Input: part model. Units: mm. Frame: model coordinates. Give positions to 0.01 mm unless a question says otherwise; leave off trailing zeros. Write each loop counter-clockwise with the first axis right and the second up, starting at its lowest first coordinate (ties: lowest second). Pieces come first, ordered by that corner, then holes.
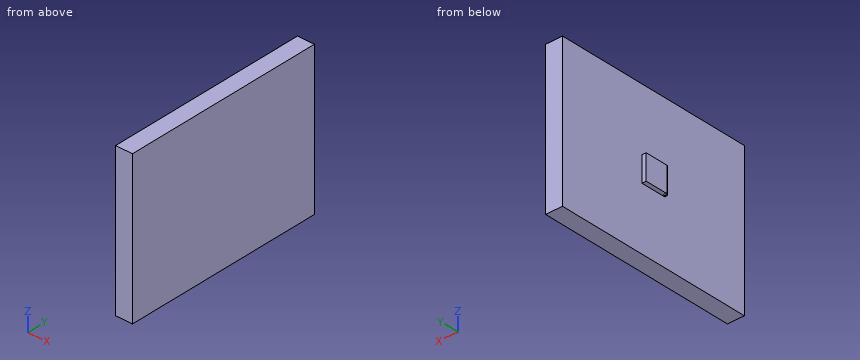
```python
from build123d import *

# Parameters (mm, degrees)
F0_W     = 304.8
F0_H     = 228.6
F1_DEPTH = 25.4
F3_DEPTH = 19.05
F5_D     = 3.175
F6_R     = 3.175


with BuildPart() as f1:
    # F0 (on Right) → F1 (new body)
    with BuildSketch(Plane.YZ):
        Rectangle(F0_W, F0_H)
    extrude(amount=F1_DEPTH)

    # F2 (on Front) → F3 (join, symmetric)
    with BuildSketch(Plane.XZ):
        Polygon((0, -19.05), (0, 19.05), (-3.175, 19.05), (-6.35, 19.05), (-6.35, -19.05), (-3.175, -19.05), align=None)
    extrude(amount=F3_DEPTH, both=True)

    # F5 (through all)
    with Locations(Plane.XY.offset(19.05)):
        with Locations((-3.175, -15.875)):
            Hole(F5_D / 2)

    # F6
    f6_edges = [f1.edges().sort_by_distance(p)[0] for p in [
        (-6.35, -19.05, 0),
    ]]
    fillet(f6_edges, radius=F6_R)


solid = f1.part
```
Q1. Pin query (flat end, axial travel): pin 1 (7 mm diameter, centred on x = -4.5, y = -9.5, fed in from +Z); pin 2 (3 mm diameter, centred on x = -4, z = 0.5, fed in from +Y); pin 3 (4 mm diameter, centred on y = -18, z = -52.5, fed in from -X). Return the tip coordinate at first contact, or that it passes through.
Q2. Material intervals for line 1 along X through (y, z) = (60.5, -9.5), sorted ascending.
Q3. Section C-C, the plane z = 100. Return the cut outline in (x, y), then the cut area to 3 significant figures.
Q4. Section B-B, the plane y = 44.5. Return the cut outline in (x, z), then the cut area to 3 significant figures.
Solutions:
1. pin 1: stops at z = 19.05
1. pin 2: stops at y = 19.05
1. pin 3: stops at x = 0
2. line 1: x = 0 to 25.4
3. outline: (0, -152.4) - (25.4, -152.4) - (25.4, 152.4) - (0, 152.4) - close
3. area: 7,740 mm2
4. outline: (0, -114.3) - (25.4, -114.3) - (25.4, 114.3) - (0, 114.3) - close
4. area: 5,810 mm2
